For this review, take the finished solid that the model builds, in its own axes (mm). A direction names the side the tool comes from. Round coordinates to 2 decimals unless told otherwise and drop trailing zeros. Order: outer loops, then holes, each group sorted by start corner. A loop starts at its lowest first (then second) coordinate and runs counter-clockwise, first axis right, second up. Notation, with made-up numbers: M 68.5,76 L 81.5,76 A25 cw 81.5,90 Z; hole C -6.5,75.5 d7. An arc over 180 degrees is marked long. Put each result on its own line as item: value.
Autodesk Inventor part; units mm, degrees
ref_plane "YZ Plane" through (0, 0, 0) normal (1, 0, 0) x (0, 1, 0)
ref_plane "XZ Plane" through (0, 0, 0) normal (0, 1, 0) x (-1, 0, 0)
ref_plane "XY Plane" through (0, 0, 0) normal (0, 0, 1) x (1, 0, 0)
sketch "Skizze1" plane through (0, 0, 0) normal (0, 1, 0) x (-1, 0, 0)
  line L0 (-6, 0) -> (1, 0) construction
  line L1 (-1.0415, 0) -> (-1.5, 2.6)
  line L2 (-1.5, 2.6) -> (-0.9176, 4.2)
  line L3 (-0.9176, 4.2) -> (-2.7176, 4.2)
  line L4 (-2.7176, 4.2) -> (-3.3, 2.6)
  line L5 (-3.3, 2.6) -> (-2.9121, 0.4)
  line L6 (-1.5, 2.6) -> (-3.3, 2.6) construction
  line L7 (-2.9121, 0.4) -> (-3.3121, 0)
  line L8 (-3.3121, 0) -> (-5, 0)
  line L9 (-5, 0) -> (-5, -0.8)
  line L10 (-5, -0.8) -> (0, -0.8)
  line L11 (0, -0.8) -> (0, 0)
  line L12 (-1.0415, 0) -> (0, 0)
  line L13 (0, -0.8) -> (0, 4.2)
  dimension "d0" = 80
  dimension "d1" = 70
  dimension "d2" = 1.8
  dimension "d3" = 2.6
  dimension "d4" = 1.6
  dimension "d21" = 45
  dimension "d22" = 0.4
  dimension "d23" = 0.8
  dimension "d24" = 10
  dimension "d26" = 6.6
revolve "Umdrehung1" add sketch "Skizze1" angle 360 about axis through (0, 0, -0.8) along (0, 0, 1)
properties part number "Druckknopf" material "Gummi, Silikon"
(1) Add section B-B on z = 2. Give the boundary of the cut face in (x, y).
A:
outline: C 0,0 d6.39; hole C 0,0 d2.79
(2) To check wall thickness, follow L1, parallel to Z at x = -2, y = -2.75; L2, parallel to Y at x = 1, z = 2.4; L3, parallel to Y at x = 0.5, z = 1.9. State the ranges of each line that lie inside material, in increasing order.
A:
L1: z = -0.8 to 0
L2: y = -3.11 to -1.07, 1.07 to 3.11
L3: y = -3.14 to -1.28, 1.28 to 3.14
(3) Add section D-D on z = 3.85. Give the boundary of the cut face in (x, y) (3 decimals), then the cut area to 3 significant figures.
A:
outline: C 0,0 d5.69; hole C 0,0 d2.09
area: 22.0 mm2
(4) Insertion check: pin 1 Ø3 at (x, z) = (1.5, 2) entering from +Y; pin 2 Ø1 at (y, z) = (0.5, 2) entering from +X; pin 3 Ø1.5 at (y, z) = (-2.5, 1) entering from +X. Each pin has a flat end and moves straight along its axis. Give the tip position at first contact, or say it passes through.
A:
pin 1: stops at y = 3.3
pin 2: stops at x = 3.26
pin 3: stops at x = 2.48
(5) For faces 1 (the face through (0, 0, -0.8)), 2 (the face through (-0.265, -1.194, 1.029)), 3 (the face through (3.3, 1.2, 0)), list the 3-axis set-ups (+Z, -Z, +X, -X, +Y, -Y) from which the entire face can be reached by the end or side of a thin tool; tool diameter is ignored.
A:
face 1: -Z, +X, -X, +Y, -Y
face 2: none
face 3: +Z
(6) Add section A-A on y = 0. Give the boundary of the cut face in (x, z).
A:
outline: M -5,-0.8 L 5,-0.8 L 5,0 L 3.31,0 L 2.91,0.4 L 3.3,2.6 L 2.72,4.2 L 0.92,4.2 L 1.5,2.6 L 1.04,0 L -1.04,0 L -1.5,2.6 L -0.92,4.2 L -2.72,4.2 L -3.3,2.6 L -2.91,0.4 L -3.31,0 L -5,0 Z
(7) Draft analysis for pull direction X (two halves, no side actions). For faces 4 (the face through (0, -1.2, 4.2)), 5 (the face through (2.883, 0.908, 1.027)), 6 (the face through (0, 0, 0)), state which applies: released by +X, released by -X, zero draft, split by the parting line, or undercut.
A:
face 4: zero draft
face 5: split by the parting line
face 6: undercut
